For this review, take the finished solid that the model builds, in its own axes (mm). A direction names the side the tool comes from. Round coordinates to 2 decimals unless told otherwise and drop trailing zeros. Loops run counter-clockwise (first coordinate to the right, second up) from the corner with the lowest first, then second, coordinate; pieces in that order, holes last.
1) Take a section at C-C (y = 40.5). State the section outline as (x, z) points, then the cut area to 3 significant figures.
2) Insertion check: pin 1 (1.5 mm diameter, centred on y = 40.5, z = 1, fed in from +X); pin 2 (1 mm diameter, centred on x = -16, z = 2.5, fed in from +Y); pin 3 (0.9 mm diameter, centred on x = -10.5, z = 2, fed in from -Y). Each pin has a flat end and moves straight along its axis. Give the tip position at first contact, or say it passes through.
3) Wall thickness on L1, parallel to X at y = 40.5, z = 0.4; L2, parallel to X at y = 42.5, z = 0.8; L3, parallel to Y at x = 4, z = 0.25: over which ranges is each line inside the solid? List them lowest first.
4) Take a section at B-B (x = -3.5). State the section outline as (y, z) points, then the cut area to 3 significant figures.
5) Tool access review of faces 1 (the flat face through (0, 39.048, 1)), 2 (the flat face through (-5, 41, 1)), 3 (the flat face through (5, 41, 1)): name each direction out of +Z, -Z, +X, -X, +Y, -Y from which nothing blocks a thin tool from reaching the whole face with its end or side.
6) Take a section at A-A (z = 2). State the section outline as (x, y) points.
Autodesk Inventor part; units mm, degrees
ref_plane "YZ Plane" through (0, 0, 0) normal (1, 0, 0) x (0, 1, 0)
ref_plane "XZ Plane" through (0, 0, 0) normal (0, 1, 0) x (-1, 0, 0)
ref_plane "XY Plane" through (0, 0, 0) normal (0, 0, 1) x (1, 0, 0)
sketch "Sketch1" plane through (0, 0, 0) normal (0, 0, 1) x (1, 0, 0)
  arc A0 (21, 42.0476) -> (-21, 42.0476) centre (0, 0) ccw
  line L0 (-5, 42.0476) -> (-5, 39.0476)
  line L1 (-5, 39.0476) -> (5, 39.0476)
  line L2 (5, 39.0476) -> (5, 42.0476)
  line L3 (-21, 42.0476) -> (-5, 42.0476)
  line L4 (5, 42.0476) -> (21, 42.0476)
  dimension "d0" = 94
  dimension "d2" = 3
  dimension "d3" = 10
  dimension "d4" = 5
  dimension "d8" = 16
  dimension "d9" = 16
extrude "Extrusion1" add sketch "Sketch1" along normal blind 3
properties part number "OpenROV_Dev_EChassis_Blinder"
Response:
1. outline: (-5, 0) - (5, 0) - (5, 3) - (-5, 3) - close
1. area: 30.0 mm2
2. pin 1: stops at x = 5
2. pin 2: stops at y = 44.37
2. pin 3: stops at y = 42.05
3. L1: x = -5 to 5
3. L2: x = -20.07 to 20.07
3. L3: y = 39.05 to 46.83
4. outline: (39.05, 0) - (46.87, 0) - (46.87, 3) - (39.05, 3) - close
4. area: 23.5 mm2
5. face 1: +Z, -Z, +X, -X, -Y
5. face 2: +Z, -Z, -X, -Y
5. face 3: +Z, -Z, +X, -Y
6. outline: (-21, 42.05) - (-5, 42.05) - (-5, 39.05) - (5, 39.05) - (5, 42.05) - (21, 42.05) arc R47 ccw to start
